Design review of the part built by this model. Coordinates are the model's own, in mm. Face numbers are marked on the shaded views. A direction names the side the tool comes from. Round coordinates to 2 decimals unless told otherwise and drop trailing zeros. Write each loop counter-clockwise with the first axis right and the second up, starting at its lowest first coordinate (ties: lowest second). Pieces come first, ordered by that corner, then holes. Notation, with made-up numbers: M -18,55.25 L 15,55.25 A12 cw 15,67.25 Z; hole C -18.75,-17 d2. An arc over 180 degrees is marked long. One line per question, with ' | ' between items. Start each with the question number.
Item 1: Add section C-C, the plane x = 0. State the section outline as (y, z) points.
Item 2: Add section D-D, the plane y = -4.25. State the section outline as (x, z) points, and give its area (3 significant figures).
Item 3: Machinability: for the marked faces 1 and 2, which of the approach directions +Z, -Z, +X, -X, +Y, -Y give a long, thin tool a straight path to every point of the face, cutting with its end or side? Answer none if there is none.
Item 4: Draft analysis for pull direction X (two halves, no side actions). For the marked faces 3, 4, 5 and 6, state which applies: released by +X, released by -X, zero draft, split by the parting line, or undercut.
Item 5: Insertion check: pin 1 Ø3 at (y, z) = (-4, 34.5) entering from -X. The pin has a flat end and moves straight along its axis. Give the tip position at first contact, or say it passes through.
Item 6: For L1, parallel to Y at x = -16.35, z = 41.5; L2, parallel to Y at x = 0, z = 11.5; L3, parallel to X at y = -7.25, z = 28, list the stretches that pass through material, from the lowest coordinate up.
Item 7: Add section A-A, the plane y = 8.75. State the section outline as (x, z) points.
```python
from build123d import *

# Parameters (mm, degrees)
SZKIC1_W                    = 28
SZKIC1_H                    = 20
SZKIC1_R                    = 6.5
DODANIE_WYCI_GNI_CIE1_DEPTH = 46
SZKIC2_W                    = 0.1
SZKIC2_H                    = 9
DODANIE_WYCI_GNI_CIE2_DEPTH = 20
WYTNIJ_WYCI_GNI_CIE1_DEPTH  = 3.3
WYTNIJ_WYCI_GNI_CIE2_DEPTH  = 3.3
SZKIC5_W                    = 9
SZKIC5_H                    = 20
SZKIC5_R                    = 2.1
DODANIE_WYCI_GNI_CIE3_DEPTH = 3.39
DODANIE_WYCI_GNI_CIE4_START = 3.39
SZKIC6_W                    = 9
SZKIC6_H                    = 20
SZKIC6_R                    = 2.1
DODANIE_WYCI_GNI_CIE4_DEPTH = 3.39
SZKIC7_W                    = 9.448344777
SZKIC7_H                    = 3
WYTNIJ_WYCI_GNI_CIE3_DEPTH  = 0.8
SZKIC8_W                    = 9
SZKIC8_H                    = 3
WYTNIJ_WYCI_GNI_CIE4_DEPTH  = 0.8


with BuildPart() as part:
    # Szkic1 → Dodanie-wyciągnięcie1 (new body)
    with BuildSketch(Plane.XY):
        Rectangle(SZKIC1_W, SZKIC1_H)
        Circle(SZKIC1_R, mode=Mode.SUBTRACT)
    extrude(amount=DODANIE_WYCI_GNI_CIE1_DEPTH)

    # Szkic2 → Dodanie-wyciągnięcie2 (add)
    with BuildSketch(Plane(origin=(0, 10, 0), x_dir=(1, 0, 0), z_dir=(0, 1, 0))):
        with Locations((-14.05, -41.5)):
            Rectangle(SZKIC2_W, SZKIC2_H)
        with Locations((14.05, -41.5)):
            Rectangle(SZKIC2_W, SZKIC2_H)
    extrude(amount=-DODANIE_WYCI_GNI_CIE2_DEPTH)

    # Szkic3 → Wytnij-wyciągnięcie1 (cut)
    with BuildSketch(Plane(origin=(14.1, 0, 0), x_dir=(0, 0, -1), z_dir=(1, 0, 0))):
        Polygon((-39.421539031, -3.6), (-37.343078062, 0), (-39.421539031, 3.6), (-46, 3.6), (-46, -3.6), align=None)
    extrude(amount=-WYTNIJ_WYCI_GNI_CIE1_DEPTH, mode=Mode.SUBTRACT)

    # Szkic4 → Wytnij-wyciągnięcie2 (cut)
    with BuildSketch(Plane.ZY.offset(14.1)):
        Polygon((41.5, 3.6), (39.421539031, 3.6), (37.343078062, 0), (39.421539031, -3.6), (46, -3.6), (46, 3.6), align=None)
    extrude(amount=-WYTNIJ_WYCI_GNI_CIE2_DEPTH, mode=Mode.SUBTRACT)

    # Szkic5 → Dodanie-wyciągnięcie3 (add)
    with BuildSketch(Plane.ZY.offset(14.1)):
        with Locations((41.5, 0)):
            Rectangle(SZKIC5_W, SZKIC5_H)
        with Locations((41.5, 0)):
            Circle(SZKIC5_R, mode=Mode.SUBTRACT)
    extrude(amount=DODANIE_WYCI_GNI_CIE3_DEPTH)

    # Szkic6 → Dodanie-wyciągnięcie4 (add)
    with BuildSketch(Plane(origin=(14.1, 0, 0), x_dir=(0, 0, -1), z_dir=(1, 0, 0)).offset(DODANIE_WYCI_GNI_CIE4_START)):
        with Locations((-41.5, 0)):
            Rectangle(SZKIC6_W, SZKIC6_H)
        with Locations(Location((-41.5, 0, 0), (0, 0, 180))):
            Circle(SZKIC6_R, mode=Mode.SUBTRACT)
    extrude(amount=-DODANIE_WYCI_GNI_CIE4_DEPTH)

    # Szkic7 → Wytnij-wyciągnięcie3 (cut)
    with BuildSketch(Plane.ZY.offset(17.49)):
        with Locations((41.724172389, 5.9)):
            Rectangle(SZKIC7_W, SZKIC7_H)
    extrude(amount=-WYTNIJ_WYCI_GNI_CIE3_DEPTH, mode=Mode.SUBTRACT)

    # Szkic8 → Wytnij-wyciągnięcie4 (cut)
    with BuildSketch(Plane(origin=(17.49, 0, 0), x_dir=(0, 0, -1), z_dir=(1, 0, 0))):
        with Locations((-41.5, 5.9)):
            Rectangle(SZKIC8_W, SZKIC8_H)
    extrude(amount=-WYTNIJ_WYCI_GNI_CIE4_DEPTH, mode=Mode.SUBTRACT)


solid = part.part
```
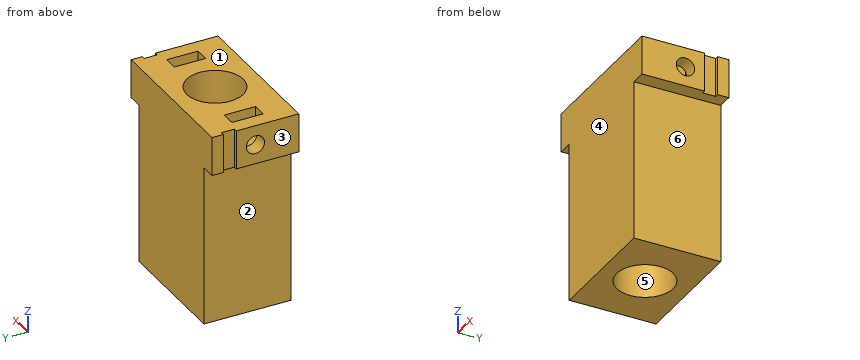
Computed values:
1) outline: M -10,0 L -6.5,0 L -6.5,46 L -10,46 Z; M 6.5,0 L 10,0 L 10,46 L 6.5,46 Z
2) outline: M -17.49,37 L -14,37 L -14,0 L -4.92,0 L -4.92,46 L -17.49,46 Z; M 4.92,0 L 14,0 L 14,37 L 17.49,37 L 17.49,46 L 4.92,46 Z | area: 898 mm^2
3) face 1: +Z, +X, -X, +Y, -Y | face 2: -Z, -X, +Y, -Y
4) face 3: released by -X | face 4: zero draft | face 5: undercut | face 6: released by +X
5) pin 1: stops at x = -14
6) L1: y = -10 to -2.1, 2.1 to 10 | L2: y = -10 to -6.5, 6.5 to 10 | L3: x = -14 to 14
7) outline: M -17.49,37 L -14,37 L -14,0 L 14,0 L 14,37 L 17.49,37 L 17.49,46 L -17.49,46 Z
